Read the model definition and answer for the solid it produces. Units are mm, in the model's axes. Coordinates: 2 decimals unless noted, no trailing zeros. Order: outer loops, then holes, each group sorted by start corner. A loop starts at its lowest first (then second) coordinate and runs counter-clockwise, first axis right, second up. Notation, with made-up numbers: (-19, 54.25) - (-2, 54.25) arc R30 cw to (-2, 83.25) - close; hole circle Ø3 at (-40, -14.75). An arc over 180 degrees is marked (long way). Write item = value, one per line.
from build123d import *

# Parameters (mm, degrees)
SKETCH1_R               = 7
SKETCH1_R_2             = 4
BOSS_EXTRUDE1_DEPTH     = 7
CUT_EXTRUDE1_REACH      = 14.124
CUT_EXTRUDE1_END_RADIUS = 7
SKETCH2_R               = 2
FILLET1_R               = 0.5
FILLET2_R               = 0.5


with BuildPart() as part:
    # Sketch1 → Boss-Extrude1 (new body)
    with BuildSketch(Plane(origin=(0, 0, 0), x_dir=(1, 0, 0), z_dir=(0, 1, 0))):
        with Locations(Location((0, 0, 0), (0, 0, 270))):
            Circle(SKETCH1_R)
        with Locations(Location((0, 0, 0), (0, 0, 270))):
            Circle(SKETCH1_R_2, mode=Mode.SUBTRACT)
    extrude(amount=BOSS_EXTRUDE1_DEPTH)

    # Cut-Extrude1: up to this cylinder (the profile starts inside it)
    cut_extrude1_end = Plane(origin=(0, 3.5, 0), z_dir=(0, -1, 0)) * Cylinder(CUT_EXTRUDE1_END_RADIUS, 43.248, mode=Mode.PRIVATE)
    # Sketch2 → Cut-Extrude1 (cut, up to the surface)
    with BuildSketch(Plane.XY, mode=Mode.PRIVATE) as cut_extrude1_sk1:
        with Locations((0, 3.5)):
            Circle(SKETCH2_R)
    cut_extrude1_tool1 = extrude(cut_extrude1_sk1.sketch, amount=-CUT_EXTRUDE1_REACH, mode=Mode.PRIVATE) & cut_extrude1_end
    add(cut_extrude1_tool1.solids().sort_by_distance((0, 3.5, 0))[0], mode=Mode.SUBTRACT)

    # Fillet1
    fillet1_edges = [part.edges().sort_by_distance(p)[0] for p in [
        (0, 0, -7),
        (0, 7, -7),
    ]]
    fillet(fillet1_edges, radius=FILLET1_R)

    # Fillet2
    fillet2_edges = [part.edges().sort_by_distance(p)[0] for p in [
        (-2, 3.5, -3.464101615),
        (0, 0, -4),
        (0, 7, -4),
    ]]
    fillet(fillet2_edges, radius=FILLET2_R)


solid = part.part
1) Flat-ended cylindrical pins translate along their axes: pin 1 Ø3 at (x, z) = (-5, -0.5) entering from -Y; pin 2 Ø3 at (x, y) = (0, 3.5) entering from -Z; pin 3 Ø1.5 at (x, y) = (-4, 5.5) entering from +Z; pin 4 Ø1 at (y, z) = (2, 4.5) entering from +X. Find the tip coordinate at first contact, or state that the pin passes through.
Returned:
pin_1 = 0
pin_2 = 3.71
pin_3 = 6.2
pin_4 = 5.74
2) Straight lines are drawn through the part: line 1 along X through (y, z) = (2.25, 0); line 2 along Z through (x, y) = (0, 3.75); line 3 along X through (y, z) = (5.25, 0.75). For each, find the intervals that lie inside material, in ascending order. Write a range as from..to.
Returned:
line_1 = -7..-4, 4..7
line_2 = 4..7
line_3 = -6.96..-3.93, 3.93..6.96
3) The part is cut by section A-A (z = 0). Determine the outline of the cut face in (x, y), and give its area (3 significant figures).
Returned:
outline = (-7, 0.5) arc R0.5 ccw to (-6.5, 0) - (-4.5, 0) arc R0.5 ccw to (-4, 0.5) - (-4, 6.5) arc R0.5 ccw to (-4.5, 7) - (-6.5, 7) arc R0.5 ccw to (-7, 6.5) - close; (4, 0.5) arc R0.5 ccw to (4.5, 0) - (6.5, 0) arc R0.5 ccw to (7, 0.5) - (7, 6.5) arc R0.5 ccw to (6.5, 7) - (4.5, 7) arc R0.5 ccw to (4, 6.5) - close
area = 41.6 mm^2
4) The part is cut by section B-B (x = 0). Count the separate pieces of the cut face and the enclosed holes in it, and give its area (3 significant figures).
Returned:
separate_pieces = 3
enclosed_holes = 0
area = 29.5 mm^2
5) Determine the mould class of faces 1 (the face through (-1.998, 3.588, -5.348)), 2 (the face through (4.42, 0, -1.54)), 3 (the face through (4.42, 7, -1.54)) for opening direction Y: pulls with the +Y half, pulls with the -Y half, needs draft (parallel to the pull), parting line crosses it, or undercut.
Returned:
face_1 = undercut
face_2 = pulls with the -Y half
face_3 = pulls with the +Y half
